Part model, mm, in its own coordinate system. A direction names the side the tool comes from. Give positions to 0.01 mm unless a question says otherwise; leave off trailing zeros. Write each loop counter-clockwise with the first axis right and the second up, starting at its lowest first coordinate (ties: lowest second). Pieces come first, ordered by that corner, then holes.
from build123d import *

# Parameters (mm, degrees)
ESQUISSE1_R                  = 16.5
EXTRUSION1_DEPTH             = 5
ESQUISSE2_R                  = 2.1
ENL_V_MAT_EXTRU_1_DEPTH      = 24.864199128
R_P_TITION_CIRCULAIRE1_COUNT = 4
ESQUISSE3_R                  = 1.25
ENL_V_MAT_EXTRU_2_DEPTH      = 24.864199128


with BuildPart() as part:
    # Esquisse1 → Extrusion1 (new body)
    with BuildSketch(Plane.XY):
        Circle(ESQUISSE1_R)
        with BuildLine():
            Line((-6, 6.020797289), (-6, -6.020797289))
            ThreePointArc((-6, -6.020797289), (0, -8.5), (6, -6.020797289))
            Line((6, -6.020797289), (6, 6.020797289))
            ThreePointArc((6, 6.020797289), (0, 8.5), (-6, 6.020797289))
        make_face(mode=Mode.SUBTRACT)
    extrude(amount=EXTRUSION1_DEPTH)

    # Esquisse2 → Enl_v. mat.-Extru.1 (cut, through all)
    with BuildSketch(Plane.XY.offset(5)):
        with Locations((0, 13)):
            Circle(ESQUISSE2_R)
    enl_v_mat_extru_1 = extrude(amount=-ENL_V_MAT_EXTRU_1_DEPTH, mode=Mode.SUBTRACT)

    # R_p_tition circulaire1: Enl_v. mat.-Extru.1 ×4 about axis
    r_p_tition_circulaire1_axis = Axis((0, 0, 0), (0, 0, 1))
    for i in range(1, R_P_TITION_CIRCULAIRE1_COUNT):
        add(enl_v_mat_extru_1.rotate(r_p_tition_circulaire1_axis, i * 360 / R_P_TITION_CIRCULAIRE1_COUNT), mode=Mode.SUBTRACT)

    # Esquisse3 → Enl_v. mat.-Extru.2 (cut, through all)
    with BuildSketch(Plane.XY.offset(5)):
        with Locations((-5.5, 0)):
            Circle(ESQUISSE3_R)
    extrude(amount=-ENL_V_MAT_EXTRU_2_DEPTH, mode=Mode.SUBTRACT)


solid = part.part
1) Drill centre lines: L1, parallel to Y at x = 0, z = 1.55; L2, parallel to Y at x = 1, z = 2.6; L3, parallel to Y at x = -13, z = 2.2. Where is each one in solid material? Low to high.
Check result:
L1: y = -16.5 to -15.1, -10.9 to -8.5, 8.5 to 10.9, 15.1 to 16.5
L2: y = -16.47 to -14.85, -11.15 to -8.44, 8.44 to 11.15, 14.85 to 16.47
L3: y = -10.16 to -2.1, 2.1 to 10.16
2) Saw through at C-C (z = 1.75). Write the cut outline in (x, y), and give its area (3 significant figures).
Check result:
outline: circle Ø33 at (0, 0); hole circle Ø4.2 at (-13, 0); hole (-6, -6.02) arc R8.5 ccw to (6, -6.02) - (6, 6.02) arc R8.5 ccw to (-6, 6.02) - (-6, 1.15) arc R1.25 ccw to (-6, -1.15) - close; hole circle Ø4.2 at (0, -13); hole circle Ø4.2 at (0, 13); hole circle Ø4.2 at (13, 0)
area: 613 mm2
3) Mould opens along X. For faces 1 (the flat face through (7, 0, 0)), 2 (the cylindrical face through (15.24, -6.32, 2.46)), 3 (the cylindrical face through (0.273, -15.082, 2.535)) say: +X half, -X half, draft (parallel to the pull), parting line (faces both ways), or undercut.
Check result:
face 1: draft
face 2: parting line
face 3: undercut
4) 3-axis set-ups, long thin cutter, end or side, ignore diameter. For faces 4 (the flat face through (7, 0, 5)), 5 (the cylindrical face through (-6.75, 0.02, 2.54)): which of +Z, -Z, +X, -X, +Y, -Y reach the whole face in a straight line?
Check result:
face 4: +Z, +X, -X, +Y, -Y
face 5: +Z, -Z
5) Saw through at D-D (y = 12). Write the cut outline in (x, z), and give its area (3 significant figures).
Check result:
outline: (-11.32, 0) - (-1.85, 0) - (-1.85, 5) - (-11.32, 5) - close; (1.85, 0) - (11.32, 0) - (11.32, 5) - (1.85, 5) - close
area: 94.8 mm2
6) Flat gauge pins, fed straight in: P1, Ø2, axis at x = 3.5, z = 4.5, coming from the +Y side; P2, Ø2.5, axis at y = 4, z = 2.5, coming from the +X side; P3, Ø1.5, axis at x = 11.5, z = 4, coming from the +Y side. Where does each tip first touch, or does it go through?
Check result:
P1: stops at y = 16.31
P2: stops at x = 16.27
P3: stops at y = 12.52
7) Saw through at B-B (y = 0). Write the cut outline in (x, z), and give its area (4 significant figures).
Check result:
outline: (-16.5, 0) - (-15.1, 0) - (-15.1, 5) - (-16.5, 5) - close; (-10.9, 0) - (-6.75, 0) - (-6.75, 5) - (-10.9, 5) - close; (6, 0) - (10.9, 0) - (10.9, 5) - (6, 5) - close; (15.1, 0) - (16.5, 0) - (16.5, 5) - (15.1, 5) - close
area: 59.25 mm2
8) Saw through at A-A (x = 0). Write the cut outline in (y, z).
Check result:
outline: (-16.5, 0) - (-15.1, 0) - (-15.1, 5) - (-16.5, 5) - close; (-10.9, 0) - (-8.5, 0) - (-8.5, 5) - (-10.9, 5) - close; (8.5, 0) - (10.9, 0) - (10.9, 5) - (8.5, 5) - close; (15.1, 0) - (16.5, 0) - (16.5, 5) - (15.1, 5) - close
